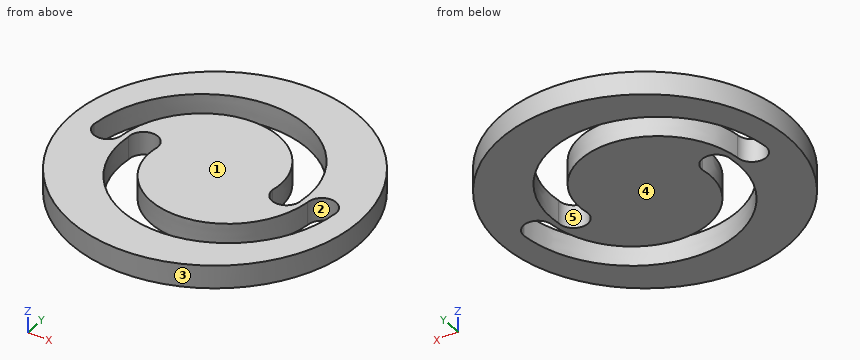
```python
from build123d import *

# Parameters (mm, degrees)
SKETCH_R        = 25
PAD_DEPTH       = 4
POCKET_DEPTH    = 5
POCKET001_DEPTH = 5


with BuildPart() as part:
    # Sketch → Pad (new body)
    with BuildSketch(Plane.XY):
        Circle(SKETCH_R)
    extrude(amount=PAD_DEPTH)

    # Sketch006 → Pocket (cut)
    with BuildSketch(Plane(origin=(0, 0, 0), x_dir=(-1, 0, 0), z_dir=(0, 0, 1))):
        with BuildLine():
            ThreePointArc((10, 0), (12.5, -2.660022), (15, 0))
            add(Edge.make_bspline(
                [(15, 0), (15.545455, 4.28399), (14.745053, 8.910699), (12.419355, 13.410338), (8.573372, 17.219141), (3.449426, 19.762244), (-2.463902, 20.569387), (-8.48908, 19.39714), (-13.890489, 16.306895), (-18.024894, 11.652452), (-20.454545, 5.997586), (-21, 0)],
                knots=[0, 0, 0, 0, 0, 0, 0, 0, 0, 0, 0, 0, 3.296908, 3.296908, 3.296908, 3.296908, 3.296908, 3.296908, 3.296908, 3.296908, 3.296908, 3.296908, 3.296908, 3.296908], degree=11))
            ThreePointArc((-21, 0), (-18.5, -2.530386), (-16, 0))
            add(Edge.make_bspline(
                [(10, 0), (10.545455, 2.855993), (10.193672, 6.054706), (8.76521, 9.282944), (6.203587, 12.133546), (2.628131, 14.160628), (-1.642606, 14.967771), (-6.119295, 14.311546), (-10.236344, 12.179501), (-13.473513, 8.796459), (-15.454545, 4.569589), (-16, 0)],
                knots=[0, 0, 0, 0, 0, 0, 0, 0, 0, 0, 0, 0, 3.296908, 3.296908, 3.296908, 3.296908, 3.296908, 3.296908, 3.296908, 3.296908, 3.296908, 3.296908, 3.296908, 3.296908], degree=11))
        make_face()
    extrude(amount=POCKET_DEPTH, mode=Mode.SUBTRACT)

    # Sketch007 → Pocket001 (cut)
    with BuildSketch(Plane.XY):
        with BuildLine():
            ThreePointArc((10, 0), (12.5, -2.660022), (15, 0))
            add(Edge.make_bspline(
                [(15, 0), (15.545455, 4.28399), (14.745053, 8.910699), (12.419355, 13.410338), (8.573372, 17.219141), (3.449426, 19.762244), (-2.463902, 20.569387), (-8.48908, 19.39714), (-13.890489, 16.306895), (-18.024894, 11.652452), (-20.454545, 5.997586), (-21, 0)],
                knots=[0, 0, 0, 0, 0, 0, 0, 0, 0, 0, 0, 0, 3.296908, 3.296908, 3.296908, 3.296908, 3.296908, 3.296908, 3.296908, 3.296908, 3.296908, 3.296908, 3.296908, 3.296908], degree=11))
            ThreePointArc((-21, 0), (-18.5, -2.530386), (-16, 0))
            add(Edge.make_bspline(
                [(10, 0), (10.545455, 2.855993), (10.193672, 6.054706), (8.76521, 9.282944), (6.203587, 12.133546), (2.628131, 14.160628), (-1.642606, 14.967771), (-6.119295, 14.311546), (-10.236344, 12.179501), (-13.473513, 8.796459), (-15.454545, 4.569589), (-16, 0)],
                knots=[0, 0, 0, 0, 0, 0, 0, 0, 0, 0, 0, 0, 3.296908, 3.296908, 3.296908, 3.296908, 3.296908, 3.296908, 3.296908, 3.296908, 3.296908, 3.296908, 3.296908, 3.296908], degree=11))
        make_face()
    extrude(amount=POCKET001_DEPTH, mode=Mode.SUBTRACT)


solid = part.part
```
CAD build for the part. Positions are in the model's coordinates, mm. Face numbers are marked on the shaded views. A direction names the side the tool comes from. Round coordinates to 2 decimals unless told otherwise and drop trailing zeros. Use CSV: the item, a comma, the result in double quotes. Start each with the question number.
1) Wall check: L1, parallel to X at y = -11, z = 2.9; L2, parallel to X at y = -7.5, z = 2.55; L3, parallel to Y at x = -9, z = 2.8. Give the ranges that are in metal, low to high. Write a range as [from, to].
2) Saw through at A-A (z = 0.65). Count the separate pieces of the cut face and the enclosed holes in it, and give its area (3 significant figures).
3) Tool access for the marked faces 4 and 5: list every direction of +Z, -Z, +X, -X, +Y, -Y with a clear straight run to the whole face (end or side of a thin tool).
4) Two-plate mould, pull along X, no slides. Class the marked faces 1, 2 and 3: pulls with the +X half, pulls with the -X half, needs draft (parallel to the pull), parting line crosses it, or undercut.
Values follow:
1,L1,"x = [-22.45, -12.17], [-5.18, 9.18], [16.56, 22.45]"
1,L2,"x = [-23.85, -14.06], [-8.55, 12.99], [18.84, 23.85]"
1,L3,"y = [-23.32, -14.34], [-6.7, 11.11], [16.67, 23.32]"
2,separate pieces,"1"
2,enclosed holes,"2"
2,area,"1,440 mm2"
3,face 4,"-Z, +X, -X, +Y, -Y"
3,face 5,"+Z, -Z"
4,face 1,"needs draft"
4,face 2,"undercut"
4,face 3,"parting line crosses it"
